Can you work these out from the model? Positions are in its coordinate system, mm. Face numbers are marked on the shaded views. A direction names the side the tool comes from. Round coordinates to 2 decimals unless told otherwise and drop trailing zeros. Order: outer loops, then holes, each group sorted by start corner. A loop starts at its lowest first (then second) coordinate and runs counter-clockwise, first axis right, second up. Notation, with made-up numbers: M 41,64.25 L 55,64.25 A22 cw 55,80.25 Z; hole C 30,80 d9. An arc over 180 degrees is marked long. One line per question, with ' | ' between items.
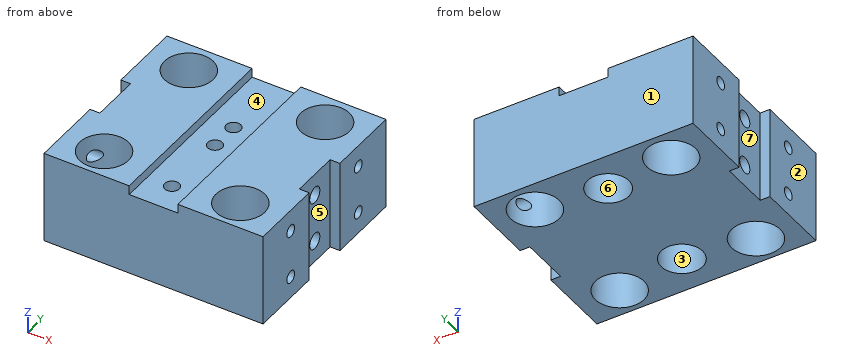
```python
from build123d import *

# Parameters (mm, degrees)
BOSS_EXTRUDE1_DEPTH   = 19
SKETCH2_W             = 10
SKETCH2_H             = 40
CUT_EXTRUDE1_DEPTH    = 1.9
SKETCH3_R             = 5
CUT_EXTRUDE2_DEPTH    = 20
SKETCH4_R             = 4.25
CUT_EXTRUDE3_DEPTH    = 10
SKETCH5_R             = 1.5
CUT_EXTRUDE4_DEPTH    = 10
M3_TAPPED_HOLE2_D     = 2.5
M3_TAPPED_HOLE2_DEPTH = 7.5
M3_TAPPED_HOLE2_TIP   = 0.751075774
M4_TAPPED_HOLE1_D     = 3.3
M4_TAPPED_HOLE1_DEPTH = 10.1
M4_TAPPED_HOLE1_TIP   = 0.991420021
M4_TAPPED_HOLE2_D     = 3.3
M4_TAPPED_HOLE2_DEPTH = 10.1
M4_TAPPED_HOLE2_TIP   = 0.991420021
M3_TAPPED_HOLE3_D     = 2.5
M3_TAPPED_HOLE3_DEPTH = 7.5
M3_TAPPED_HOLE3_TIP   = 0.751075774


with BuildPart() as part:
    # Sketch1 → Boss-Extrude1 (new body)
    with BuildSketch(Plane.XY):
        Polygon((-19.512195122, -12.317073171), (-19.512195122, -27.317073171), (25.487804878, -27.317073171), (25.487804878, -12.317073171), (23.487804878, -12.317073171), (23.487804878, -2.317073171), (25.487804878, -2.317073171), (25.487804878, 12.682926829), (-19.512195122, 12.682926829), (-19.512195122, -2.317073171), (-17.512195122, -2.317073171), (-17.512195122, -12.317073171), align=None)
    extrude(amount=BOSS_EXTRUDE1_DEPTH)

    # Sketch2 → Cut-Extrude1 (cut)
    with BuildSketch(Plane.XY.offset(19)):
        with Locations((2.987804878, -7.317073171)):
            Rectangle(SKETCH2_W, SKETCH2_H)
    extrude(amount=-CUT_EXTRUDE1_DEPTH, mode=Mode.SUBTRACT)

    # Sketch3 → Cut-Extrude2 (cut, through all)
    with BuildSketch(Plane.XY.offset(19)):
        with Locations((-11.012195122, 6.337375375)):
            Circle(SKETCH3_R)
        with Locations((16.987804878, 6.337375375)):
            Circle(SKETCH3_R)
        with Locations((-11.012195122, -21.251537573)):
            Circle(SKETCH3_R)
        with Locations((16.987804878, -21.251537573)):
            Circle(SKETCH3_R)
    extrude(amount=-CUT_EXTRUDE2_DEPTH, mode=Mode.SUBTRACT)

    # Sketch4 → Cut-Extrude3 (cut)
    with BuildSketch(Plane(origin=(0, 0, 0), x_dir=(-1, 0, 0), z_dir=(0, 0, -1))):
        with Locations((-2.987804878, -19.317073171)):
            Circle(SKETCH4_R)
        with Locations((-2.987804878, 4.682926829)):
            Circle(SKETCH4_R)
    extrude(amount=-CUT_EXTRUDE3_DEPTH, mode=Mode.SUBTRACT)

    # Sketch5 → Cut-Extrude4 (cut)
    with BuildSketch(Plane.XY.offset(17.1)):
        with Locations((2.987804878, -1.317073171)):
            Circle(SKETCH5_R)
        with Locations((2.987804878, -7.317073171)):
            Circle(SKETCH5_R)
        with Locations((2.987804878, -21.317073171)):
            Circle(SKETCH5_R)
    extrude(amount=-CUT_EXTRUDE4_DEPTH, mode=Mode.SUBTRACT)

    # M3 Tapped Hole2
    with Locations(Plane.ZY.offset(19.512195122)):
        with Locations((14.5, 3.682926829), (4.5, 3.682926829), (14.5, -18.317073171), (4.5, -18.317073171)):
            Hole(M3_TAPPED_HOLE2_D / 2, depth=M3_TAPPED_HOLE2_DEPTH)
            with Locations((0, 0, -(M3_TAPPED_HOLE2_DEPTH + M3_TAPPED_HOLE2_TIP / 2))):  # 118° drill point
                Cone(0, M3_TAPPED_HOLE2_D / 2, M3_TAPPED_HOLE2_TIP, mode=Mode.SUBTRACT)

    # M4 Tapped Hole1
    with Locations(Plane.ZY.offset(17.512195122)):
        with Locations((14.5, -7.317073171), (4.5, -7.317073171)):
            Hole(M4_TAPPED_HOLE1_D / 2, depth=M4_TAPPED_HOLE1_DEPTH)
            with Locations((0, 0, -(M4_TAPPED_HOLE1_DEPTH + M4_TAPPED_HOLE1_TIP / 2))):  # 118° drill point
                Cone(0, M4_TAPPED_HOLE1_D / 2, M4_TAPPED_HOLE1_TIP, mode=Mode.SUBTRACT)

    # M4 Tapped Hole2
    with Locations(Plane(origin=(23.487804878, 0, 0), x_dir=(0, 0, -1), z_dir=(1, 0, 0))):
        with Locations((-14.5, -7.317073171), (-4.5, -7.317073171)):
            Hole(M4_TAPPED_HOLE2_D / 2, depth=M4_TAPPED_HOLE2_DEPTH)
            with Locations((0, 0, -(M4_TAPPED_HOLE2_DEPTH + M4_TAPPED_HOLE2_TIP / 2))):  # 118° drill point
                Cone(0, M4_TAPPED_HOLE2_D / 2, M4_TAPPED_HOLE2_TIP, mode=Mode.SUBTRACT)

    # M3 Tapped Hole3
    with Locations(Plane(origin=(25.487804878, 0, 0), x_dir=(0, 0, -1), z_dir=(1, 0, 0))):
        with Locations((-14.5, -18.317073171), (-4.5, -18.317073171), (-4.5, 3.682926829), (-14.5, 3.682926829)):
            Hole(M3_TAPPED_HOLE3_D / 2, depth=M3_TAPPED_HOLE3_DEPTH)
            with Locations((0, 0, -(M3_TAPPED_HOLE3_DEPTH + M3_TAPPED_HOLE3_TIP / 2))):  # 118° drill point
                Cone(0, M3_TAPPED_HOLE3_D / 2, M3_TAPPED_HOLE3_TIP, mode=Mode.SUBTRACT)


solid = part.part
```
(1) If we section it at B-B on y = -3.5: Please give me the cut outline in (x, z), plus the area to 3 significant figures.
Final values:
outline: M -17.51,0 L 23.49,0 L 23.49,19 L 7.99,19 L 7.99,17.1 L -2.01,17.1 L -2.01,19 L -17.51,19 Z | area: 760 mm^2
(2) If we section it at C-C on z = 11.25: Please give me the cut outline in (x, y), plus the area to 3 significant figures.
Final values:
outline: M -19.51,-27.32 L 25.49,-27.32 L 25.49,-12.32 L 23.49,-12.32 L 23.49,-2.32 L 25.49,-2.32 L 25.49,12.68 L -19.51,12.68 L -19.51,-2.32 L -17.51,-2.32 L -17.51,-12.32 L -19.51,-12.32 Z; hole C -11.01,-21.25 d10; hole C -11.01,6.34 d10; hole C 2.99,-21.32 d3; hole C 2.99,-7.32 d3; hole C 2.99,-1.32 d3; hole C 16.99,-21.25 d10; hole C 16.99,6.34 d10 | area: 1,420 mm^2
(3) On a 3-axis mill with a long thin cutter (end or side, diameter ignored), from which of +Z, -Z, +X, -X, +Y, -Y can I reach the whole of each face in a straight line? I mean the marked faces 4, 5, 6 and 7. Say none if no direction works.
Final values:
face 4: +Z, +Y, -Y | face 5: +Z, -Z, +X | face 6: -Z | face 7: +Z, -Z, -X
(4) If we section it at A-A on x = 16.5: Please give me the cut outline in (y, z), plus the area to 3 significant figures.
Final values:
outline: M -27.32,0 L -26.23,0 L -26.23,19 L -27.32,19 Z; M -16.28,0 L 1.36,0 L 1.36,19 L -16.28,19 Z; M 11.31,0 L 12.68,0 L 12.68,19 L 11.31,19 Z; hole C -7.32,4.5 d3.3; hole C -7.32,14.5 d3.3 | area: 365 mm^2
(5) Thinking about a two-plate mould opening in Y: for the marked faces 1, 2 and 3, which applies, released by +Y, released by -Y, zero draft, split by the parting line, or undercut?
Final values:
face 1: released by +Y | face 2: zero draft | face 3: undercut
(6) Will these pins go through, and if not, where does the flat tip stop? pin 1 Ø1.5 at (y, z) = (3.68, 4.5) entering from +X; pin 2 Ø0.9 at (x, y) = (3.5, -1.5) entering from +Z; pin 3 Ø8 at (x, y) = (2.5, -0.5) entering from +Z; pin 4 Ø5 at (x, y) = (7, -21.5) entering from -Z.
Final values:
pin 1: x = 13.33 | pin 2: z = 7.1 | pin 3: z = 17.1 | pin 4: z = 0
(7) Please list where these lines run through material, in increasing order: probe 1 along Y at (x, z) = (-17.65, 4.5); probe 2 along Z at (x, y) = (18, -7.5); probe 3 along X at (y, z) = (9.5, 7.75). Write a range as [from, to].
Final values:
probe 1: [-27.32, -19.57], [-17.07, -12.32], [-2.32, 2.43], [4.93, 12.68] | probe 2: [0, 2.86], [6.14, 12.86], [16.14, 19] | probe 3: [-19.51, -14.88], [-7.14, 13.12], [20.86, 25.49]
(8) If we section it at D-D on y = -22: Please give me the cut outline in (x, z).
Final values:
outline: M -19.51,0 L -15.96,0 L -15.96,19 L -19.51,19 Z; M -6.07,0 L -0.31,0 L -0.31,10 L 1.65,10 L 1.65,17.1 L -2.01,17.1 L -2.01,19 L -6.07,19 Z; M 4.32,10 L 6.28,10 L 6.28,0 L 12.04,0 L 12.04,19 L 7.99,19 L 7.99,17.1 L 4.32,17.1 Z; M 21.93,0 L 25.49,0 L 25.49,19 L 21.93,19 Z
